Part print with two shaded views. Sizes in mm from the minimum x, y, z corner. A direction names the side the tool comes from. Give positions to 0.01 mm unless a question says otherwise; leave off trailing zeros. Write each loop counter-clockwise with the first axis right and the second up, starting at its lowest first coordinate (ties: lowest second). Pieces come first, ordered by that corner, then holes.
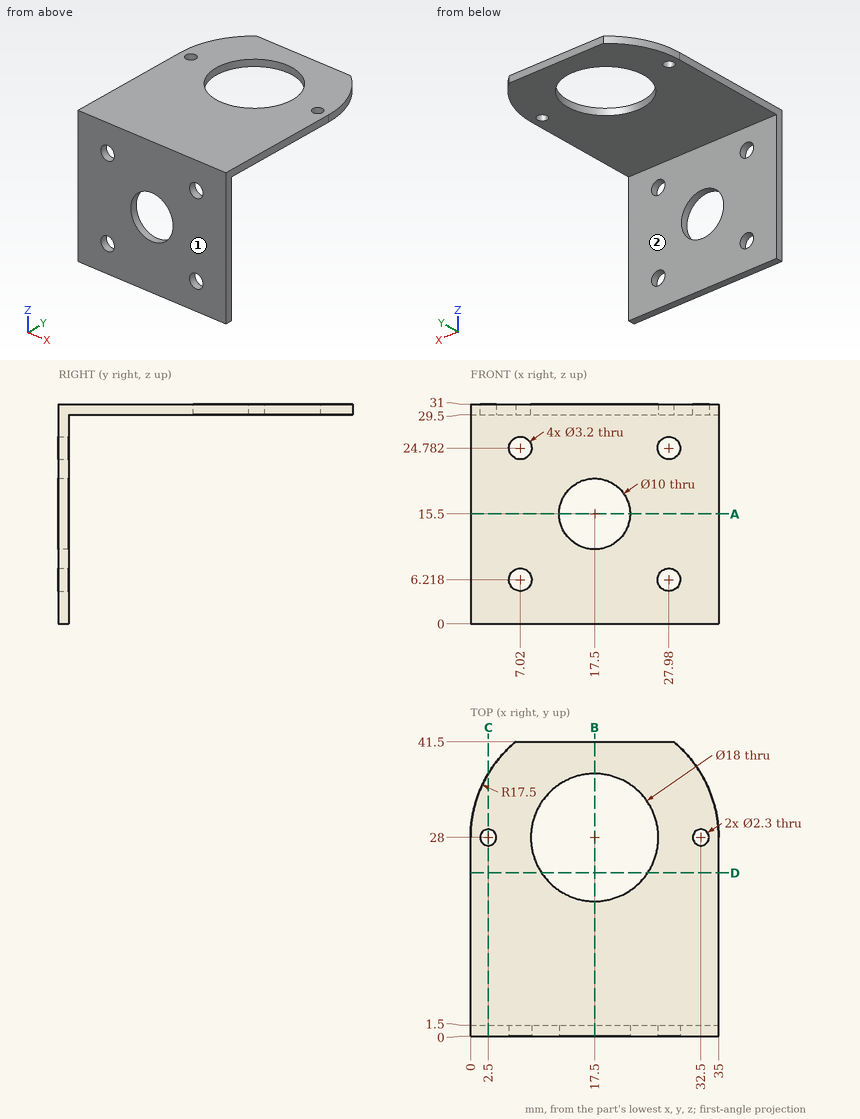
(1) Probe line 1 (Y direction, x = 23.5, z = 16); line 2 (Z direction, x = 19.5, y = 5.5); line 3 (Y direction, x = 32, z = 30) (1 decimal). List the from-to ranges inside material, lowest first.
(2) Saw through at D-D, the plane y = 23. List the corners of the cut face in (x, z).
(3) Drop flat-ended pins along their axis: pin 1 (10 mm diameter, centred on x = 27.5, z = 19, fed in from +Y); pin 2 (10.5 mm diameter, centred on x = 21.5, y = 24.5, fed in from -Z). Give the stop position or say it passes through.
(4) Saw through at C-C, the plane x = 2.5. List the corners of the cut face in (y, z).
(5) Saw through at A-A, the plane z = 15.5. List the corners of the cut face in (x, y).
(6) Saw through at B-B, the plane x = 17.5. List the corners of the cut face in (y, z).
(7) 3-axis set-ups, long thin cutter, end or side, ignore diameter. For the marked faces 1 and 2: which of +Z, -Z, +X, -X, +Y, -Y reach the whole face in a straight line?
Computed values:
1. line 1: y = 0 to 1.5
1. line 2: z = 29.5 to 31
1. line 3: y = 0 to 27, 29 to 37.8
2. outline: (0, 29.5) - (10.02, 29.5) - (10.02, 31) - (0, 31) - close; (24.98, 29.5) - (35, 29.5) - (35, 31) - (24.98, 31) - close
3. pin 1: stops at y = 1.5
3. pin 2: stops at z = 29.5
4. outline: (0, 0) - (1.5, 0) - (1.5, 29.5) - (26.85, 29.5) - (26.85, 31) - (0, 31) - close; (29.15, 29.5) - (37.01, 29.5) - (37.01, 31) - (29.15, 31) - close
5. outline: (0, 0) - (12.5, 0) - (12.5, 1.5) - (0, 1.5) - close; (22.5, 0) - (35, 0) - (35, 1.5) - (22.5, 1.5) - close
6. outline: (0, 0) - (1.5, 0) - (1.5, 10.5) - (0, 10.5) - close; (0, 20.5) - (1.5, 20.5) - (1.5, 29.5) - (19, 29.5) - (19, 31) - (0, 31) - close; (37, 29.5) - (41.5, 29.5) - (41.5, 31) - (37, 31) - close
7. face 1: +Z, -Z, +X, -X, -Y
7. face 2: -Z, +X, -X, +Y
